Source: CAD feature listing. Evaluate the final solid. Frame: model axes, mm. Face numbers are marked on the shaded views. Round coordinates to 2 decimals unless told otherwise and drop trailing zeros. Order: outer loops, then holes, each group sorted by start corner. A loop starts at its lowest first (then second) coordinate and runs counter-clockwise, first axis right, second up. Notation, with made-up numbers: M 80,42 L 106,42 A19 ccw 106,75 Z; hole C -40,63.25 d3. An arc over 180 degrees is marked long. Use one line per item in the form item = value. Start each with the question number.
Q1. Pull-direction query (Z, two-part tool) for the marked faces 1 and 2; classes: pulls with the +Z half, pulls with the -Z half, needs draft (parallel to the pull), parting line crosses it, or undercut.
Q2. Section A-A (y = 2.5). Return the cut outline in (x, z) (3 decimals).
Q3. Material intervals for probe 1 along X at (y, z) = (0.85, -7.62) (3 decimals); probe 2 along Z at (x, y) = (-10.5, 2.8) (3 decimals); probe 3 along Y at (x, z) = (19.5, 2.25), sorted ascending.
Q4. Section D-D (x = -2). Return the cut outline in (y, z) (3 decimals).
Q5. Section B-B (z = 7.62). Return the cut outline in (x, y) (3 decimals).
Q6. Contact query for flat-ended pins moving along their axis: pin 1 (1 mm diameter, centred on y = 2, z = -7, fed in from -X); pin 2 (1.5 mm diameter, centred on x = -20.32, z = 7.62, fed in from +Y); pin 3 (0.6 mm diameter, centred on y = 3, z = -7.5, fed in from +X). Output: stop coordinate, or through.
Q7. Section C-C (x = -20.32). Return the cut outline in (y, z) (3 decimals), plus the area to 3 significant figures.
from build123d import *

# Parameters (mm, degrees)
SKETCH2_W                                  = 43.18
SKETCH2_H                                  = 17.78
BOSS_EXTRUDE1_DEPTH                        = 1.27
SKETCH3_R                                  = 0.635
CUT_EXTRUDE1_DEPTH                         = 24.383179852
MIRROR1_AT_THE_SECOND_PLANE_COPY_1_SKETC_R = 0.635
MIRROR1_AT_THE_SECOND_PLANE_COPY_1_DEPTH   = 24.383179852
SKETCH4_W                                  = 37.381103683
SKETCH4_H                                  = 2.016737313
BOSS_EXTRUDE2_DEPTH                        = 2.54


with BuildPart() as part:
    # Sketch2 → Boss-Extrude1 (new body)
    with BuildSketch(Plane(origin=(0, 0, 0), x_dir=(1, 0, 0), z_dir=(0, 1, 0))):
        Rectangle(SKETCH2_W, SKETCH2_H)
    extrude(amount=BOSS_EXTRUDE1_DEPTH)

    # Sketch3 → Cut-Extrude1 (cut, symmetric)
    with BuildSketch(Plane(origin=(0, 1.27, 0), x_dir=(1, 0, 0), z_dir=(0, 1, 0))):
        with Locations(Location((-20.32, 7.62, 0), (0, 0, 270))):
            Circle(SKETCH3_R)
    cut_extrude1 = extrude(amount=CUT_EXTRUDE1_DEPTH, both=True, mode=Mode.SUBTRACT)

    # Mirror1: Cut-Extrude1 across plane
    add(cut_extrude1.mirror(Plane(origin=(0, 0, 0), x_dir=(0, 0, 1), z_dir=(1, 0, 0))), mode=Mode.SUBTRACT)

    # Mirror1 at the second plane: Cut-Extrude1 across plane
    add(cut_extrude1.mirror(Plane.XY), mode=Mode.SUBTRACT)

    # Mirror1 at the second plane copy 1 sketc → Mirror1 at the second plane copy 1 (cut, symmetric)
    with BuildSketch(Plane(origin=(0, 1.27, 0), x_dir=(-1, 0, 0), z_dir=(0, 1, 0))):
        with Locations(Location((-20.32, 7.62, 0), (0, 0, 270))):
            Circle(MIRROR1_AT_THE_SECOND_PLANE_COPY_1_SKETC_R)
    extrude(amount=MIRROR1_AT_THE_SECOND_PLANE_COPY_1_DEPTH, both=True, mode=Mode.SUBTRACT)

    # Sketch4 → Boss-Extrude2 (add)
    with BuildSketch(Plane(origin=(0, 1.27, 0), x_dir=(1, 0, 0), z_dir=(0, 1, 0))):
        with Locations((0.021963045, -7.246631344)):
            Rectangle(SKETCH4_W, SKETCH4_H)
    boss_extrude2 = extrude(amount=BOSS_EXTRUDE2_DEPTH)

    # Mirror2: Boss-Extrude2 across plane
    add(boss_extrude2.mirror(Plane.XY))


solid = part.part
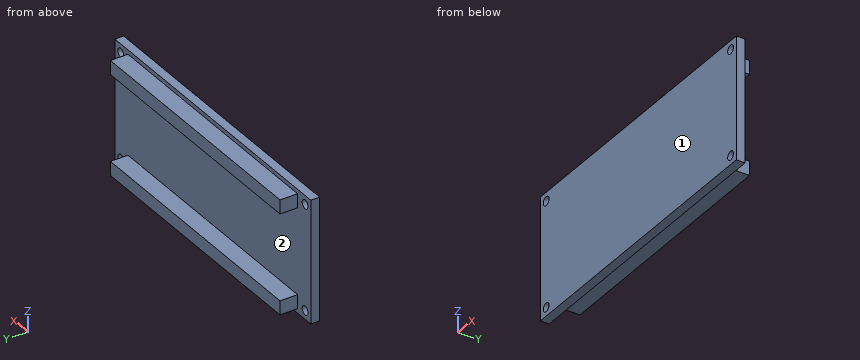
Results list:
q1.face_1 = needs draft
q1.face_2 = undercut
q2.outline = M -18.669,-8.255 L 18.713,-8.255 L 18.713,-6.238 L -18.669,-6.238 Z; M -18.669,6.238 L 18.713,6.238 L 18.713,8.255 L -18.669,8.255 Z
q3.probe_1 = -21.59 to -20.955, -19.685 to 19.685, 20.955 to 21.59
q3.probe_2 = -8.255 to -6.238, 6.238 to 8.255
q3.probe_3 = 0 to 1.27
q4.outline = M 0,-8.89 L 1.27,-8.89 L 1.27,-8.255 L 3.81,-8.255 L 3.81,-6.238 L 1.27,-6.238 L 1.27,6.238 L 3.81,6.238 L 3.81,8.255 L 1.27,8.255 L 1.27,8.89 L 0,8.89 Z
q5.outline = M -21.59,0 L -20.955,0 L -20.955,1.27 L -21.59,1.27 Z; M -19.685,0 L 19.685,0 L 19.685,1.27 L 18.713,1.27 L 18.713,3.81 L -18.669,3.81 L -18.669,1.27 L -19.685,1.27 Z; M 20.955,0 L 21.59,0 L 21.59,1.27 L 20.955,1.27 Z
q6.pin_1 = -18.67
q6.pin_2 = 1.27
q6.pin_3 = 18.71
q7.outline = M 0,-8.89 L 1.27,-8.89 L 1.27,-8.255 L 0,-8.255 Z; M 0,-6.985 L 1.27,-6.985 L 1.27,6.985 L 0,6.985 Z; M 0,8.255 L 1.27,8.255 L 1.27,8.89 L 0,8.89 Z
q7.area = 19.4 mm2
